from build123d import *

# Parameters (mm, degrees)
BOSS_EXTRUDE1_DEPTH     = 12.5
SKETCH2_W               = 12.5
SKETCH2_H               = 2
BOSS_EXTRUDE2_DEPTH     = 6
SKETCH3_R               = 1.5
CUT_EXTRUDE1_DEPTH      = 32.713927878
CUT_EXTRUDE1_DEPTH_BACK = 16.499999831
SKETCH5_W               = 8.5
SKETCH5_H               = 8.5
CUT_EXTRUDE2_DEPTH      = 26.999999831


with BuildPart() as part:
    # Sketch1 → Boss-Extrude1 (new body)
    with BuildSketch(Plane.XY):
        with BuildLine():
            ThreePointArc((8, 17), (7.694207367, 19.190701486), (6.80020675, 21.213927878))
            Line((6.80020675, 21.213927878), (4.814885895, 18.847914617))
            ThreePointArc((4.814885895, 18.847914617), (4.953505298, 18.180283222), (5, 17.5))
            Line((5, 17.5), (5, -17.5))
            ThreePointArc((5, -17.5), (0, -22.5), (-5, -17.5))
            Line((-5, -17.5), (-5, 17.5))
            Line((-5, 17.5), (-7.984359711, 17.5))
            ThreePointArc((-7.984359711, 17.5), (-7.996088972, 17.250122279), (-8, 17))
            Line((-8, 17), (-8, -17.999999662))
            ThreePointArc((-8, -17.999999662), (-1.69e-07, -25.999999831), (8, -18))
            Line((8, -18), (8, 17))
        make_face()
    extrude(amount=BOSS_EXTRUDE1_DEPTH)

    # Sketch2 → Boss-Extrude2 (add)
    with BuildSketch(Plane(origin=(8, 0, 0), x_dir=(0, 0, -1), z_dir=(1, 0, 0))):
        with Locations((-6.25, -11.5)):
            Rectangle(SKETCH2_W, SKETCH2_H)
        with Locations((-6.25, -6.5)):
            Rectangle(SKETCH2_W, SKETCH2_H)
    extrude(amount=BOSS_EXTRUDE2_DEPTH)

    # Sketch3 → Cut-Extrude1 (cut, two sides)
    with BuildSketch(Plane(origin=(0, -10.5, 0), x_dir=(1, 0, 0), z_dir=(0, 1, 0))) as cut_extrude1_sk:
        with Locations((11, -3)):
            Circle(SKETCH3_R)
        with Locations((11, -9.5)):
            Circle(SKETCH3_R)
    extrude(amount=CUT_EXTRUDE1_DEPTH, mode=Mode.SUBTRACT)
    extrude(cut_extrude1_sk.sketch, amount=-CUT_EXTRUDE1_DEPTH_BACK, mode=Mode.SUBTRACT)

    # Sketch5 → Cut-Extrude2 (cut, through all)
    with BuildSketch(Plane(origin=(0, 0, 0), x_dir=(1, 0, 0), z_dir=(0, 1, 0))):
        with Locations((0, -6.25)):
            Rectangle(SKETCH5_W, SKETCH5_H)
    extrude(amount=-CUT_EXTRUDE2_DEPTH, mode=Mode.SUBTRACT)


solid = part.part
The model under review builds one solid part; all positions refer to its coordinate system, in mm. A direction names the side the tool comes from. Round coordinates to 2 decimals unless told otherwise and drop trailing zeros. Write each loop counter-clockwise with the first axis right and the second up, starting at its lowest first coordinate (ties: lowest second). Pieces come first, ordered by that corner, then holes. Notation, with made-up numbers: M -22.5,31 L 25.5,31 A37 cw 25.5,69 Z; hole C 80.25,32.25 d5. An arc over 180 degrees is marked long. Use a Markdown table: item, result. Add a question column.
Q1. We need section B-B, the plane x = 0. State the section outline as (y, z) points, plus the area to 3 significant figures.
Q2. We need section D-D, the plane z = 5.75. State the section outline as (x, y) points.
Q3. Insertion check: pin 1 (0.9 mm diameter, centred on x = -6.5, z = 3.5, fed in from +Y); pin 2 (3.5 mm diameter, centred on x = 11, z = 3, fed in from +Y); pin 3 (3 mm diameter, centred on x = 11, z = 9, fed in from -Y). Each pin has a flat end and moves straight along its axis. Give the tip position at first contact, or say it passes through.
Q4. We need section C-C, the plane z = 9.5. Count the separate pieces of the cut face and the enclosed holes in it, plus the area to 3 significant figures.
Q5. Machinability: for faces 4 (the face through (4.25, -22, 6)), 5 (the face through (8, -15, 6)), 6 (the face through (8, -9, 6)), 7 (the face through (11, -5.5, 6)), which of the approach directions +Z, -Z, +X, -X, +Y, -Y give a long, thin tool a straight path to every point of the face, cutting with its end or side? Answer none if there is none.
Q6. The part is to be moulded in two halves that separate along X. For faces 1 (the face through (8, 6, 6)), 2 (the face through (-8, 0, 6)), 3 (the face through (5, 0, 6)), say which applies: pulls with the +X half, pulls with the -X half, needs draft (parallel to the pull), parting line crosses it, or undercut.
Q7. To check wall thickness, follow line 1 (X direction, y = -11.6, z = 9.5); line 2 (X direction, y = 13.5, z = 5.25); line 3 (Z direction, x = 11, y = -11.2). State the ranges of each line that lie inside material, in increasing order.
Q8. We need section A-A, the plane y = -13. State the section outline as (x, z) points, plus the area to 3 significant figures.
Findings below:
| question | item | result |
|---|---|---|
| 1 | outline | M -26,0 L -22.5,0 L -22.5,2 L -26,2 Z; M -26,10.5 L -22.5,10.5 L -22.5,12.5 L -26,12.5 Z |
| 1 | area | 14.0 mm² |
| 2 | outline | M -8,-18 A8 ccw -4.25,-24.78 L -4.25,-20.13 A5 cw -5,-17.5 L -5,17.5 L -7.98,17.5 A8 ccw -8,17 Z; M 4.25,-24.78 A8 ccw 8,-18 L 8,-12.5 L 14,-12.5 L 14,-10.5 L 8,-10.5 L 8,-7.5 L 14,-7.5 L 14,-5.5 L 8,-5.5 L 8,17 A8 ccw 6.8,21.21 L 4.81,18.85 A5 cw 5,17.5 L 5,-17.5 A5 cw 4.25,-20.13 Z |
| 3 | pin 1 | stops at y = 17.5 |
| 3 | pin 2 | stops at y = -5.5 |
| 3 | pin 3 | stops at y = -12.5 |
| 4 | separate pieces | 4 |
| 4 | enclosed holes | 0 |
| 4 | area | 267 mm² |
| 5 | face 4 | +Y, -Y |
| 5 | face 5 | +Z, -Z, +X, -Y |
| 5 | face 6 | +Z, -Z, +X |
| 5 | face 7 | +Z, -Z, +X, +Y |
| 6 | face 1 | pulls with the +X half |
| 6 | face 2 | pulls with the -X half |
| 6 | face 3 | undercut |
| 7 | line 1 | x = -8 to -5, 5 to 9.5, 12.5 to 14 |
| 7 | line 2 | x = -8 to -5, 5 to 8 |
| 7 | line 3 | z = 0 to 1.5, 4.5 to 8, 11 to 12.5 |
| 8 | outline | M -8,0 L -5,0 L -5,12.5 L -8,12.5 Z; M 5,0 L 8,0 L 8,12.5 L 5,12.5 Z |
| 8 | area | 75.0 mm² |
